```python
from build123d import *

# Parameters (mm, degrees)
ESQUISSE1_W             = 4.2
ESQUISSE1_H             = 5
ESQUISSE2_R             = 2.5
BOSS_EXTRU_1_DEPTH      = 20
ENL_V_MAT_EXTRU_1_DEPTH = 3
CHANFREIN1_SIZE         = 0.5
CONG_1_R                = 0.5


with BuildPart() as part:
    # Esquisse1 → Révolution1 (revolve)
    with BuildSketch(Plane.XY, mode=Mode.PRIVATE) as r_volution1_sk:
        with Locations((2.1, 2.5)):
            Rectangle(ESQUISSE1_W, ESQUISSE1_H)
    revolve(r_volution1_sk.sketch.rotate(Axis((0, 5, 0), (0, -1, 0)), 270), axis=Axis((0, 5, 0), (0, -1, 0)))

    # Esquisse2 → Boss.-Extru.1 (add)
    with BuildSketch(Plane.XZ):
        with Locations(Location((0, 0, 0), (0, 0, 270))):
            Circle(ESQUISSE2_R)
    extrude(amount=BOSS_EXTRU_1_DEPTH)

    # Esquisse3 → Enlèv. mat.-Extru.1 (cut)
    with BuildSketch(Plane(origin=(0, 5, 0), x_dir=(-1, 0, 0), z_dir=(0, 1, 0))):
        Polygon((1.183568052, 2.05), (-1.183568052, 2.05), (-2.367136104, 0), (-1.183568052, -2.05), (1.183568052, -2.05), (2.367136104, 0), align=None)
    extrude(amount=-ENL_V_MAT_EXTRU_1_DEPTH, mode=Mode.SUBTRACT)

    # Chanfrein1
    chanfrein1_edges = [part.edges().sort_by_distance(p)[0] for p in [
        (0, -20, 2.5),
    ]]
    chamfer(chanfrein1_edges, length=CHANFREIN1_SIZE)

    # Congé1
    cong_1_edges = [part.edges().sort_by_distance(p)[0] for p in [
        (0, 5, 4.2),
    ]]
    fillet(cong_1_edges, radius=CONG_1_R)


solid = part.part
```
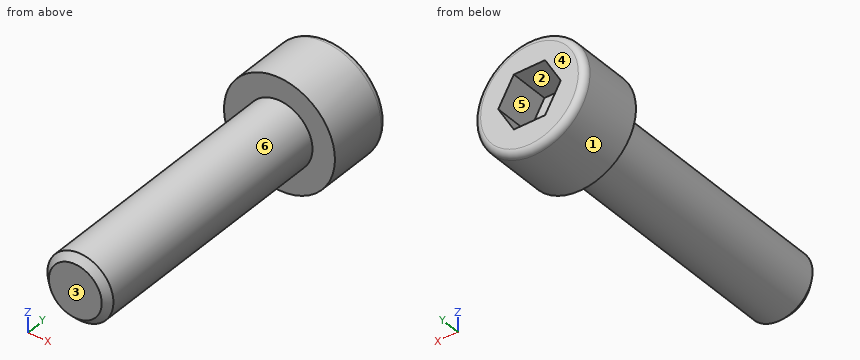
The listing builds one solid part. Answer for the finished solid, in the listing's coordinates (mm). Face numbers are marked on the shaded views. A direction names the side the tool comes from. Round coordinates to 2 decimals unless told otherwise and drop trailing zeros. Loops run counter-clockwise (first coordinate to the right, second up) from the corner with the lowest first, then second, coordinate; pieces in that order, holes last.
1) A cutting plane is placed at A-A on x = 0. Determine the outline of the cut face in (y, z).
Outcome:
outline: (-20, -2) - (-19.5, -2.5) - (0, -2.5) - (0, -4.2) - (4.5, -4.2) arc R0.5 ccw to (5, -3.7) - (5, -2.05) - (2, -2.05) - (2, 2.05) - (5, 2.05) - (5, 3.7) arc R0.5 ccw to (4.5, 4.2) - (0, 4.2) - (0, 2.5) - (-19.5, 2.5) - (-20, 2) - close
2) Consider line 1 (Y direction, x = -2.5, z = -2.25); line 2 (X direction, y = -14.5, z = 1.5). Determine where each line is inside the solid, lowest interval first.
Outcome:
line 1: y = 0 to 5
line 2: x = -2 to 2
3) A cutting plane is placed at B-B on y = -9.5. Determine the outline of the cut face in (x, z).
Outcome:
outline: circle Ø5 at (0, 0)
4) For a pull along Z with two mould halves and no side action, classify the marked faces 1, 2 and 3 as released by +Z, released by -Z, zero draft, split by the parting line, or undercut.
Outcome:
face 1: split by the parting line
face 2: undercut
face 3: zero draft
5) For the marked faces 4, 5 and 6, determine the directions among +Z, -Z, +X, -X, +Y, -Y from which every point of the face is accessible in a straight line to the end or side of a thin tool.
Outcome:
face 4: +Z, -Z, +X, -X, +Y
face 5: +Y
face 6: -Y
6) Given P1, Ø1.5, axis at y = -13, z = -2.5, coming from the +X side; P2, Ø1, axis at x = 1.5, y = -12, coming from the +Z side; P3, Ø4, axis at y = -13.5, z = -2.5, coming from the +X side, each flat-ended and moving along its own axis, determine where each tip first touches the part or whether it passes through.
Outcome:
P1: stops at x = 1.79
P2: stops at z = 2.29
P3: stops at x = 2.45
